```python
from build123d import *

# Parameters (mm, degrees)
BOSS_EXTRUDE2_DEPTH          = 431.8
CUT_EXTRUDE3_DEPTH           = 127
SKETCH7_R                    = 6.3881
CUT_EXTRUDE4_DEPTH           = 438.372816156
F_10_0_1935_DIAMETER_HOLE3_D = 4.9149


with BuildPart() as part:
    # Sketch3 → Boss-Extrude2 (new body)
    with BuildSketch(Plane.XY):
        Polygon((0, 0), (0, 49.2125), (-1.5875, 49.2125), (-1.5875, -1.5875), (49.2125, -1.5875), (49.2125, 0), align=None)
    extrude(amount=BOSS_EXTRUDE2_DEPTH)

    # Sketch6 → Cut-Extrude3 (cut)
    with BuildSketch(Plane(origin=(0, 0, 0), x_dir=(0, 0, -1), z_dir=(1, 0, 0))):
        with BuildLine():
            Line((-174.752, 39.1795), (-47.752, 39.1795))
            ThreePointArc((-47.752, 39.1795), (-33.401, 24.8285), (-47.752, 10.4775))
            Line((-47.752, 10.4775), (-174.752, 10.4775))
            ThreePointArc((-174.752, 10.4775), (-189.103, 24.8285), (-174.752, 39.1795))
        make_face()
    extrude(amount=-CUT_EXTRUDE3_DEPTH, mode=Mode.SUBTRACT)

    # Sketch7 → Cut-Extrude4 (cut, through all)
    with BuildSketch(Plane(origin=(0, 0, 0), x_dir=(0, 0, -1), z_dir=(1, 0, 0))):
        with Locations(Location((-402.336, 24.773594829, 0), (0, 0, 90))):
            Circle(SKETCH7_R)
    extrude(amount=-CUT_EXTRUDE4_DEPTH, mode=Mode.SUBTRACT)

    # #10 (0.1935) Diameter Hole3 (through all)
    with Locations(Plane(origin=(0, 0, 0), x_dir=(0, 0, -1), z_dir=(1, 0, 0))):
        with Locations((-177.8, 44.2595), (-144.526, 44.2595), (-111.252, 44.2595), (-177.8, 5.3975), (-144.526, 5.3975), (-111.252, 5.3975), (-77.978, 44.2595), (-44.704, 44.2595), (-44.704, 5.3975), (-77.978, 5.3975)):
            Hole(F_10_0_1935_DIAMETER_HOLE3_D / 2)


solid = part.part
```
Could you check a few things on this model? Use its own coordinates, in mm. A direction names the side the tool comes from. Give positions to 0.01 mm unless a question says otherwise; leave off trailing zeros. Loops run counter-clockwise (first coordinate to the right, second up) from the corner with the lowest first, then second, coordinate; pieces in that order, holes last. Notation, with made-up numbers: (-4, -17.5) -> (20, -17.5) arc R21 cw to (20, 7.5) -> close; hole circle Ø10 at (-40, 13.5). An arc over 180 degrees is marked (long way). Put each result on its own line as item: value.
(1) For faces 1 (the face through (0, 24, 213)), 2 (the face through (-0.8, 24.5, 189.1)), 3 (the face through (-1, 13, 431.8)), which set-ups out of +Z, -Z, +X, -X, +Y, -Y let a thin tool reach every point of the face, with its end or its side?
Computed:
face 1: +Z, -Z, +X, +Y
face 2: +X, -X
face 3: +Z, +X, -X, +Y, -Y
(2) Imagine slicing it at C-C on x = 13.5. Write out the boundary of the cut face in (y, z), plus the area to 3 significant figures.
Computed:
outline: (-1.59, 0) -> (0, 0) -> (0, 431.8) -> (-1.59, 431.8) -> close
area: 685 mm^2
(3) Imagine slicing it at B-B on z = 365. Write out the boundary of the cut face in (x, y).
Computed:
outline: (-1.59, -1.59) -> (49.21, -1.59) -> (49.21, 0) -> (0, 0) -> (0, 49.21) -> (-1.59, 49.21) -> close
(4) Imagine slicing it at A-A on y = 27. Write out the boundary of the cut face in (x, z), plus the area to 3 significant figures.
Computed:
outline: (-1.59, 0) -> (0, 0) -> (0, 33.57) -> (-1.59, 33.57) -> close; (-1.59, 188.94) -> (0, 188.94) -> (0, 396.35) -> (-1.59, 396.35) -> close; (-1.59, 408.32) -> (0, 408.32) -> (0, 431.8) -> (-1.59, 431.8) -> close
area: 420 mm^2
(5) Thinking about a two-plate mould opening in Z: for faces 4 (the face through (-1, 13, 0)), 5 (the face through (-0.78, 23.94, 408.67)), 6 (the face through (23, -1.588, 213)), which applies, pulls with the +Z half, pulls with the -Z half, needs draft (parallel to the pull), parting line crosses it, or undercut?
Computed:
face 4: pulls with the -Z half
face 5: undercut
face 6: needs draft
(6) Please list where this line runs through material, in increasing order: probe 1 along Y at (x, z) = (24, 366.5). Write a range as [from, to].
Computed:
probe 1: [-1.59, 0]
(7) I'm going to push flat-ended pins straight in: pin 1 Ø24.5 at (x, z) = (14.5, 287) entering from +Y; pin 2 Ø4 at (y, z) = (5.4, 111.25) entering from +X; pin 3 Ø8 at (y, z) = (5.4, 177.8) entering from +X. Where does each tip first touch, or does it pass through?
Computed:
pin 1: y = 0
pin 2: through
pin 3: x = 0
